Read the model definition and answer for the solid it produces. Units are mm, in the model's axes. A direction names the side the tool comes from. Coordinates: 2 decimals unless noted, no trailing zeros. Loops run counter-clockwise (first coordinate to the right, second up) from the corner with the lowest first, then second, coordinate; pieces in that order, holes last. Notation, with made-up numbers: M 75,41 L 123,41 A7 ccw 123,50 Z; hole C 37,-3.75 d8. An arc over 180 degrees is marked long. Put each result on its own line as item: value.
from build123d import *

# Parameters (mm, degrees)
BOSS_EXTRUDE1_DEPTH = 8
SKETCH3_R           = 6
BOSS_EXTRUDE2_DEPTH = 75


with BuildPart() as part:
    # Sketch1 → Boss-Extrude1 (new body)
    with BuildSketch(Plane(origin=(0, 0, 0), x_dir=(1, 0, 0), z_dir=(0, 1, 0))):
        Polygon((5.196152423, 9), (-5.196152423, 9), (-10.392304845, 0), (-5.196152423, -9), (5.196152423, -9), (10.392304845, 0), align=None)
    extrude(amount=BOSS_EXTRUDE1_DEPTH)

    # Sketch2 → Cut-Revolve1 (revolve, cut)
    with BuildSketch(Plane.XY):
        Polygon((-10.392304845, 0), (-9, 0), (-10.392304845, 0.803847577), align=None)
        Polygon((-10.392304845, 8), (-9, 8), (-10.392304845, 7.196152423), align=None)
    revolve(axis=Axis((0, 55, 0), (0, -1, 0)), mode=Mode.SUBTRACT)

    # Sketch3 → Boss-Extrude2 (add)
    with BuildSketch(Plane.XZ):
        Circle(SKETCH3_R)
    extrude(amount=BOSS_EXTRUDE2_DEPTH)


solid = part.part
1) Straight lines are drawn through the part: line 1 (Y direction, x = 3.75, z = -8); line 2 (X direction, y = -35.5, z = -3); line 3 (Z direction, x = -4, y = -68). For each, find the intervals that lie inside material, in ascending order. Write a range as [from, to].
Answer list:
line 1: y = [0, 8]
line 2: x = [-5.2, 5.2]
line 3: z = [-4.47, 4.47]
2) Given pin 1 Ø1 at (x, z) = (4, -6.5) entering from -Y; pin 2 Ø3 at (y, z) = (-38, 1.5) entering from -X; pin 3 Ø12 at (x, y) = (7, -20.5) entering from +Z, each flat-ended and moving along its own axis, determine where each tip first touches the part or whether it passes through.
Answer list:
pin 1: stops at y = 0
pin 2: stops at x = -6
pin 3: stops at z = 5.92
3) Which of the six approach directions +Z, -Z, +X, -X, +Y, -Y give full straight-line access (tool end or side, diameter ignored) to faces 1 (the conical face through (4.649, 7.805, -8.099)), 2 (the flat face through (2, 0, 6))?
Answer list:
face 1: -Z, +X, +Y
face 2: -Y
4) Find section A-A, the plane y = -39. Write down the section's boundary in (x, z), plus the area to 3 significant figures.
Answer list:
outline: C 0,0 d12
area: 113 mm^2
